from build123d import *

# Parameters (mm, degrees)
F1_DEPTH = 10
F2_DEPTH = 6
F3_DEPTH = 5
F4_R     = 5
F5_R     = 3


with BuildPart() as f1:
    # F0 (on Top) → F1 (new body)
    with BuildSketch(Plane.XY):
        Polygon((-12, -12), (-12, 12), (12, 12), (12, 15), (-15, 15), (-15, -12), align=None)
        Polygon((12, 12), (-12, 12), (-12, -12), (-10, -12), (-10, 10), (12, 10), align=None)
        Polygon((-15, 15), (12, 15), (12, 18), (-18, 18), (-18, -12), (-15, -12), align=None)
    extrude(amount=-F1_DEPTH)

    # F0 (on Top) → F2 (join)
    with BuildSketch(Plane.XY):
        Polygon((-15, 15), (12, 15), (12, 18), (-18, 18), (-18, -12), (-15, -12), align=None)
    extrude(amount=F2_DEPTH)

    # F0 (on Top) → F3 (join)
    with BuildSketch(Plane.XY):
        Polygon((12, 12), (-12, 12), (-12, -12), (-10, -12), (-10, 10), (12, 10), align=None)
    extrude(amount=F3_DEPTH)

    # F4
    f4_edges = [f1.edges().sort_by_distance(p)[0] for p in [
        (-10, 10, -2.5),
    ]]
    fillet(f4_edges, radius=F4_R)

    # F5
    f5_edges = [f1.edges().sort_by_distance(p)[0] for p in [
        (-18, 18, -2),
    ]]
    fillet(f5_edges, radius=F5_R)


solid = f1.part
Work out the finished part from the listing and answer in its coordinate system (mm). A direction names the side the tool comes from. Round coordinates to 2 decimals unless told otherwise and drop trailing zeros. Write each loop counter-clockwise with the first axis right and the second up, starting at its lowest first coordinate (ties: lowest second). Pieces come first, ordered by that corner, then holes.
1) A cutting plane is placed at C-C (z = -1.25). Give the vertices of the cut face in (x, y), plus the area to 3 significant figures.
2) A tool of negligible diameter and unlimited length cuts with its end or side. For faces 1 (the flat face through (-12, 0, 2)), 2 (the flat face through (0, 12, 2)), 3 (the flat face through (-10, -4, -3)), 4 (the flat face through (-10, 7, 5)), from which of +Z, -Z, +X, -X, +Y, -Y can it reach the whole face along a straight path? Write none if from no direction.
3) A cutting plane is placed at D-D (x = -13.25). Give the vertices of the cut face in (y, z).
4) A cutting plane is placed at B-B (x = 0). Give the vertices of the cut face in (y, z).
5) Straight lines are drawn through the part: line 1 (X direction, y = -9.25, z = 0.5); line 2 (Z direction, x = -3, y = 13.25); line 3 (Y direction, x = -11.5, z = 1). For each, find the intervals that lie inside material, in ascending order.
6) A cutting plane is placed at A-A (z = 3.75). Give the vertices of the cut face in (x, y).
7) Given pin 1 Ø7.5 at (x, z) = (7, -4.5) entering from -Y; pin 2 Ø12 at (x, y) = (-4, 5) entering from +Z; pin 3 Ø3 at (y, z) = (0.5, 3) entering from +X, each flat-ended and moving along its own axis, determine where each tip first touches the part or whether it passes through.
8) The mould has two halves that part along X. Classify faces 5 (the flat face through (-18, 2, -2)), 6 (the flat face through (-1, 18, -2)), 7 (the flat face through (-15, 1, 3)): pulls with the +X half, pulls with the -X half, needs draft (parallel to the pull), parting line crosses it, or undercut.
Completed:
1. outline: (-18, -12) - (-10, -12) - (-10, 5) arc R5 cw to (-5, 10) - (12, 10) - (12, 18) - (-15, 18) arc R3 ccw to (-18, 15) - close
1. area: 419 mm2
2. face 1: +Z, -Y
2. face 2: +Z, +X
2. face 3: +Z, -Z, +X, -Y
2. face 4: +Z, +X, -Y
3. outline: (-12, -10) - (18, -10) - (18, 6) - (15, 6) - (15, 0) - (-12, 0) - close
4. outline: (10, -10) - (18, -10) - (18, 6) - (15, 6) - (15, 0) - (12, 0) - (12, 5) - (10, 5) - close
5. line 1: x = -18 to -15, -12 to -10
5. line 2: z = -10 to 0
5. line 3: y = -12 to 12, 15 to 18
6. outline: (-18, -12) - (-15, -12) - (-15, 15) - (12, 15) - (12, 18) - (-15, 18) arc R3 ccw to (-18, 15) - close; (-12, -12) - (-10, -12) - (-10, 5) arc R5 cw to (-5, 10) - (12, 10) - (12, 12) - (-12, 12) - close
7. pin 1: stops at y = 10
7. pin 2: stops at z = 5
7. pin 3: stops at x = -10
8. face 5: pulls with the -X half
8. face 6: needs draft
8. face 7: undercut
